Check sheet for the modelled part. Datum: model origin and axes. Units: mm. Coordinates: 2 decimals unless noted, no trailing zeros. Write each loop counter-clockwise with the first axis right and the second up, starting at its lowest first coordinate (ties: lowest second). Pieces come first, ordered by that corner, then holes. Notation, with made-up numbers: (8.25, -37) -> (12.25, -37) arc R16 ccw to (12.25, -24) -> close; hole circle Ø8 at (58.25, 28). An arc over 180 degrees is marked (long way). Put each result on its own line as item: value.
```python
from build123d import *

# Parameters (mm, degrees)
SKETCH1_W           = 1080
SKETCH1_H           = 492
BOSS_EXTRUDE1_DEPTH = 2
SKETCH4_W           = 1104
SKETCH4_H           = 504.01209321
SKETCH4_W_2         = 1080
SKETCH4_H_2         = 492
BOSS_EXTRUDE3_DEPTH = 4
SKETCH5_W           = 1080
SKETCH5_H           = 134
CUT_EXTRUDE2_DEPTH  = 4
LPATTERN2_COUNT     = 3
LPATTERN2_PITCH     = 164


with BuildPart() as part:
    # Sketch1 → Boss-Extrude1 (new body)
    with BuildSketch(Plane(origin=(0, 0, 0), x_dir=(1, 0, 0), z_dir=(0, 1, 0))):
        Rectangle(SKETCH1_W, SKETCH1_H)
    extrude(amount=BOSS_EXTRUDE1_DEPTH)

    # Sketch4 → Boss-Extrude3 (add)
    with BuildSketch(Plane(origin=(0, 0, 0), x_dir=(1, 0, 0), z_dir=(0, 1, 0))):
        Rectangle(SKETCH4_W, SKETCH4_H)
        Rectangle(SKETCH4_W_2, SKETCH4_H_2, mode=Mode.SUBTRACT)
    extrude(amount=BOSS_EXTRUDE3_DEPTH)

    # Sketch5 → Cut-Extrude2 (cut)
    with BuildSketch(Plane(origin=(0, 2, 0), x_dir=(1, 0, 0), z_dir=(0, 1, 0))):
        with Locations((0, 164)):
            Rectangle(SKETCH5_W, SKETCH5_H)
    cut_extrude2 = extrude(amount=-CUT_EXTRUDE2_DEPTH, mode=Mode.SUBTRACT)

    # LPattern2: Cut-Extrude2 ×3
    with Locations(*[(0, 0, i * LPATTERN2_PITCH) for i in range(1, LPATTERN2_COUNT)]):
        add(cut_extrude2, mode=Mode.SUBTRACT)


solid = part.part
```
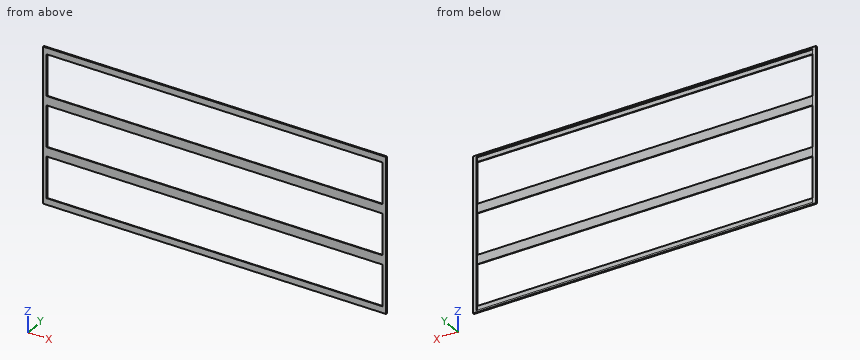
Q1. Depth check by flat-ended pin: P1, Ø15, axis at x = -12.5, z = 79, coming from the +Y side. Enter the tip coordinate at first touch or a pass-through.
Recorded:
P1: stops at y = 2
Q2. Cross-section at D-D (z = 81). Record the cut outline in (x, y).
Recorded:
outline: (-552, 0) -> (552, 0) -> (552, 4) -> (540, 4) -> (540, 2) -> (-540, 2) -> (-540, 4) -> (-552, 4) -> close
Q3. Material ranges on line 1 along Z through (x, y) = (-149, 0.65); line 2 along Z through (x, y) = (-225, 3.4); line 3 along X through (y, z) = (3.4, -110.5), recorded low to high.
Recorded:
line 1: z = -252.01 to -231, -97 to -67, 67 to 97, 231 to 252.01
line 2: z = -252.01 to -246, 246 to 252.01
line 3: x = -552 to -540, 540 to 552
Q4. Cross-section at A-A (x = 430.5). Record the cut outline in (y, z).
Recorded:
outline: (0, -252.01) -> (4, -252.01) -> (4, -246) -> (2, -246) -> (2, -231) -> (0, -231) -> close; (0, -97) -> (2, -97) -> (2, -67) -> (0, -67) -> close; (0, 67) -> (2, 67) -> (2, 97) -> (0, 97) -> close; (0, 231) -> (2, 231) -> (2, 246) -> (4, 246) -> (4, 252.01) -> (0, 252.01) -> close
Q5. Cross-section at B-B (y = 2.75). Record the cut outline in (x, z), plus the area to 3 significant figures.
Recorded:
outline: (-552, -252.01) -> (552, -252.01) -> (552, 252.01) -> (-552, 252.01) -> close; hole (-540, -246) -> (540, -246) -> (540, 246) -> (-540, 246) -> close
area: 25,100 mm2
Q6. Cross-section at C-C (z = 206). Record the cut outline in (x, y), plus the area to 3 significant figures.
Recorded:
outline: (-552, 0) -> (-540, 0) -> (-540, 4) -> (-552, 4) -> close; (540, 0) -> (552, 0) -> (552, 4) -> (540, 4) -> close
area: 96.0 mm2
